```python
from build123d import *

# Parameters (mm, degrees)
SKETCH_1_W                       = 75
SKETCH_1_H                       = 80
SM_BASE_FLANGE_1_DEPTH           = 5
SM_EDGE_FLANGE_1_STRIP_W         = 21.4732
SM_EDGE_FLANGE_1_STRIP_H         = 5
SM_EDGE_FLANGE_1_STRIP_CUT_DEPTH = 75
SM_EDGE_FLANGE_1_DEPTH           = 75
EXTRUDE_1_DEPTH                  = 2.5
CUT_EXTRUDE_1_DEPTH              = 129.16005618
FILLET_1_R                       = 5
FILLET_2_R                       = 10
CUT_EXTRUDE_2_DEPTH              = 128.401923062
CUT_EXTRUDE_3_DEPTH              = 143.324453275


# Sheet-metal steps are written as plain solids
with BuildPart() as part:
    # Sketch 1 → 基体-法兰1 (new body)
    with BuildSketch(Plane.XY):
        Rectangle(SKETCH_1_W, SKETCH_1_H)
    extrude(amount=-SM_BASE_FLANGE_1_DEPTH)

    # 边线-法兰1 strip (across the edge) → 边线-法兰1 strip cut (cut)
    with BuildSketch(Plane(origin=(37.5, 40, 0), x_dir=(0, -1, 0), z_dir=(-1, 0, 0))):
        with Locations((-5, -2.5)):
            Rectangle(SM_EDGE_FLANGE_1_STRIP_W, SM_EDGE_FLANGE_1_STRIP_H)
    extrude(amount=SM_EDGE_FLANGE_1_STRIP_CUT_DEPTH, mode=Mode.SUBTRACT)

    # 边线-法兰1 section (across the edge) → 边线-法兰1 (add)
    with BuildSketch(Plane(origin=(37.5, 40, 0), x_dir=(0, -1, 0), z_dir=(-1, 0, 0))):
        with BuildLine():
            Line((0, 0.7366), (0, 115))
            Line((0, 115), (5, 115))
            Line((5, 115), (5, 0.7366))
            ThreePointArc((5, 0.7366), (5.215745145, 0.215745145), (5.7366, 0))
            Line((5.7366, 0), (5.7366, -5))
            ThreePointArc((5.7366, -5), (1.680211239, -3.319788761), (0, 0.7366))
        make_face()
    extrude(amount=SM_EDGE_FLANGE_1_DEPTH)

    # 草图9 → 凸台-拉伸1 (add, symmetric)
    with BuildSketch(Plane(origin=(0, 0, 0), x_dir=(0, 0, -1), z_dir=(1, 0, 0))):
        with BuildLine():
            Line((-115, 35), (-115, 25))
            Line((-115, 25), (-10, -40))
            Line((-10, -40), (0, -40))
            Line((0, -40), (0, 34.2634))
            ThreePointArc((0, 34.2634), (-0.215745145, 34.784254855), (-0.7366, 35))
            Line((-0.7366, 35), (-115, 35))
        make_face()
    extrude(amount=EXTRUDE_1_DEPTH, both=True)

    # 草图10 → 切除-拉伸1 (cut, through all)
    with BuildSketch(Plane(origin=(2.5, 0, 0), x_dir=(0, 0, -1), z_dir=(1, 0, 0))):
        Polygon((-10, 25), (-96.001401484, 25), (-10, -28.238962824), align=None)
    extrude(amount=-CUT_EXTRUDE_1_DEPTH, mode=Mode.SUBTRACT)

    # 圆角1
    fillet_1_edges = [part.edges().sort_by_distance(p)[0] for p in [
        (0, 25, 115),
        (0, -40, 10),
        (0, 25, 10),
        (0, -28.238962824, 10),
        (0, 25, 96.001401484),
    ]]
    fillet(fillet_1_edges, radius=FILLET_1_R)

    # 圆角2
    fillet_2_edges = [part.edges().sort_by_distance(p)[0] for p in [
        (37.5, 37.5, 115),
        (-37.5, 37.5, 115),
        (37.5, -40, -2.5),
        (-37.5, -40, -2.5),
    ]]
    fillet(fillet_2_edges, radius=FILLET_2_R)

    # 草图11 → 切除-拉伸2 (cut, through all)
    with BuildSketch(Plane.XY):
        with BuildLine():
            Line((-16.7, -9), (-16.7, -21))
            ThreePointArc((-16.7, -21), (-20, -24.3), (-23.3, -21))
            Line((-23.3, -21), (-23.3, -9))
            ThreePointArc((-23.3, -9), (-20, -5.7), (-16.7, -9))
        make_face()
        with BuildLine():
            Line((-23.3, 9), (-23.3, 21))
            ThreePointArc((-23.3, 21), (-20, 24.3), (-16.7, 21))
            Line((-16.7, 21), (-16.7, 9))
            ThreePointArc((-16.7, 9), (-20, 5.7), (-23.3, 9))
        make_face()
        with BuildLine():
            Line((16.7, 9), (16.7, 21))
            ThreePointArc((16.7, 21), (20, 24.3), (23.3, 21))
            Line((23.3, 21), (23.3, 9))
            ThreePointArc((23.3, 9), (20, 5.7), (16.7, 9))
        make_face()
        with BuildLine():
            Line((23.3, -9), (23.3, -21))
            ThreePointArc((23.3, -21), (20, -24.3), (16.7, -21))
            Line((16.7, -21), (16.7, -9))
            ThreePointArc((16.7, -9), (20, -5.7), (23.3, -9))
        make_face()
    extrude(amount=-CUT_EXTRUDE_2_DEPTH, mode=Mode.SUBTRACT)

    # 草图12 → 切除-拉伸3 (cut, through all)
    with BuildSketch(Plane.XZ.offset(-35)):
        with BuildLine():
            Line((-16.7, 83.5), (-16.7, 71.5))
            ThreePointArc((-16.7, 71.5), (-20, 68.2), (-23.3, 71.5))
            Line((-23.3, 71.5), (-23.3, 83.5))
            ThreePointArc((-23.3, 83.5), (-20, 86.8), (-16.7, 83.5))
        make_face()
        with BuildLine():
            Line((23.3, 83.5), (23.3, 71.5))
            ThreePointArc((23.3, 71.5), (20, 68.2), (16.7, 71.5))
            Line((16.7, 71.5), (16.7, 83.5))
            ThreePointArc((16.7, 83.5), (20, 86.8), (23.3, 83.5))
        make_face()
        with BuildLine():
            Line((16.7, 31.5), (16.7, 43.5))
            ThreePointArc((16.7, 43.5), (20, 46.8), (23.3, 43.5))
            Line((23.3, 43.5), (23.3, 31.5))
            ThreePointArc((23.3, 31.5), (20, 28.2), (16.7, 31.5))
        make_face()
        with BuildLine():
            Line((-23.3, 31.5), (-23.3, 43.5))
            ThreePointArc((-23.3, 43.5), (-20, 46.8), (-16.7, 43.5))
            Line((-16.7, 43.5), (-16.7, 31.5))
            ThreePointArc((-16.7, 31.5), (-20, 28.2), (-23.3, 31.5))
        make_face()
    extrude(amount=-CUT_EXTRUDE_3_DEPTH, mode=Mode.SUBTRACT)


solid = part.part
```
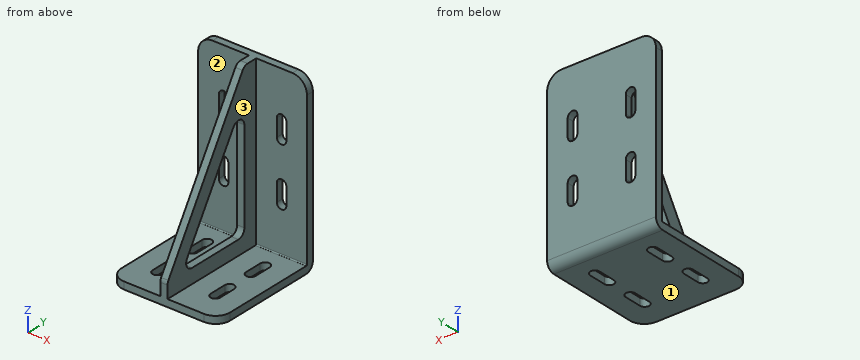
Could you check a few things on this model? Use its own coordinates, in mm. Face numbers are marked on the shaded views. A direction names the side the tool comes from. Round coordinates to 2 decimals unless told otherwise and drop trailing zeros. Write each loop counter-clockwise with the first axis right and the second up, starting at its lowest first coordinate (ties: lowest second). Pieces come first, ordered by that corner, then holes.
(1) Suppose I cut it at D-D on y = 7.5. Write out the boundary of the cut face in (x, z).
Findings below:
outline: (-37.5, -5) - (-22.94, -5) - (-22.94, 0) - (-37.5, 0) - close; (-17.06, -5) - (17.06, -5) - (17.06, 0) - (2.5, 0) - (2.5, 10) - (-2.5, 10) - (-2.5, 0) - (-17.06, 0) - close; (-2.5, 67.73) - (2.5, 67.73) - (2.5, 86.73) - (-2.5, 86.73) - close; (22.94, -5) - (37.5, -5) - (37.5, 0) - (22.94, 0) - close
(2) For pin 1 (12 mm diameter, centred on y = 13.5, z = 90, fed in from -X); pin 2 (5 mm diameter, centred on x = 29.5, z = 83, fed in from -Y); pin 3 (5.5 mm diameter, centred on x = -0.5, z = 60.5, fed in from -Y), each with a flat end and sliding along its axis, tell me the tip position at first contact or that it passes through.
Findings below:
pin 1: stops at x = -2.5
pin 2: stops at y = 35
pin 3: stops at y = -10.44
(3) Which directions (+Z, -Z, +X, -X, +Y, -Y) give clear straight access to the entire face, cutting with the end or side of a thin tool? Please do the marked faces 1, 2 and 3.
Findings below:
face 1: -Z, +X, -X, +Y, -Y
face 2: +Z, -X, -Y
face 3: +Z, +X, -Y
(4) Suppose I cut it at B-B on z = 76.5. Write out the boundary of the cut face in (x, y), and give its area (3 significant figures).
Findings below:
outline: (-37.5, 35) - (-23.3, 35) - (-23.3, 40) - (-37.5, 40) - close; (-16.7, 35) - (-2.5, 35) - (-2.5, 25) - (2.5, 25) - (2.5, 35) - (16.7, 35) - (16.7, 40) - (-16.7, 40) - close; (-2.5, 1.17) - (2.5, 1.17) - (2.5, 12.93) - (-2.5, 12.93) - close; (23.3, 35) - (37.5, 35) - (37.5, 40) - (23.3, 40) - close
area: 418 mm2
(5) If I drill on probe 1 along Z at (x, y) = (-22, 31.5); probe 2 along Y at (x, z) = (-28, 67); probe 3 along X at (y, z) = (31.5, 75.5), over which ranges is the centre line in solid material (lowest first)?
Findings below:
probe 1: z = -5 to 0
probe 2: y = 35 to 40
probe 3: x = -2.5 to 2.5
(6) Suppose I cut it at C-C on z = 58.5. Write out the boundary of the cut face in (x, y), and give its area (3 significant figures).
Findings below:
outline: (-37.5, 35) - (-2.5, 35) - (-2.5, 25) - (2.5, 25) - (2.5, 35) - (37.5, 35) - (37.5, 40) - (-37.5, 40) - close; (-2.5, -9.98) - (2.5, -9.98) - (2.5, 1.78) - (-2.5, 1.78) - close
area: 484 mm2
(7) Suppose I cut it at A-A on x = -20. Write out the boundary of the cut face in (y, z), and give its area (3 significant figures).
Findings below:
outline: (-40, -5) - (-24.3, -5) - (-24.3, 0) - (-40, 0) - close; (-5.7, -5) - (5.7, -5) - (5.7, 0) - (-5.7, 0) - close; (24.3, -5) - (34.26, -5) arc R5.74 ccw to (40, 0.74) - (40, 28.2) - (35, 28.2) - (35, 0.74) arc R0.74 cw to (34.26, 0) - (24.3, 0) - close; (35, 46.8) - (40, 46.8) - (40, 68.2) - (35, 68.2) - close; (35, 86.8) - (40, 86.8) - (40, 115) - (35, 115) - close
area: 596 mm2
